```python
from build123d import *

# Parameters (mm, degrees)
BOSS_EXTRUDE1_DEPTH = 40
SKETCH3_R           = 2.5
CUT_EXTRUDE1_DEPTH  = 10
FILLET3_R           = 20


with BuildPart() as part:
    # Sketch1 → Boss-Extrude1 (new body)
    with BuildSketch(Plane.XY):
        Polygon((125.008360384, 233.626853351), (-36.649714989, -46.373146649), (413.350285011, -46.373146649), (413.350285011, 233.626853351), align=None)
        Polygon((393.350285011, 193.626853351), (393.350285011, -16.373146649), (3.764803854, -16.373146649), (125.008360384, 193.626853351), align=None, mode=Mode.SUBTRACT)
    extrude(amount=BOSS_EXTRUDE1_DEPTH)

    # Sketch3 → Cut-Extrude1 (cut)
    with BuildSketch(Plane(origin=(0, 0, 0), x_dir=(-1, 0, 0), z_dir=(0, 0, -1))):
        with Locations((-180.923528507, 226.126853351)):
            Circle(SKETCH3_R)
        with Locations((-200.923528507, 211.126853351)):
            Circle(SKETCH3_R)
        with Locations((-220.923528507, 226.126853351)):
            Circle(SKETCH3_R)
    cut_extrude1 = extrude(amount=-CUT_EXTRUDE1_DEPTH, mode=Mode.SUBTRACT)

    # Mirror1: Cut-Extrude1 across plane
    add(cut_extrude1.mirror(Plane(origin=(264.955285011, 0, 0), x_dir=(0, 0, 1), z_dir=(1, 0, 0))), mode=Mode.SUBTRACT)

    # Fillet3
    fillet3_edges = [part.edges().sort_by_distance(p)[0] for p in [
        (393.350285011, 193.626853351, 20),
        (125.008360384, 193.626853351, 20),
        (3.764803854, -16.373146649, 20),
        (393.350285011, -16.373146649, 20),
        (-36.649714989, -46.373146649, 20),
        (125.008360384, 233.626853351, 20),
        (413.350285011, 233.626853351, 20),
        (413.350285011, -46.373146649, 20),
    ]]
    fillet(fillet3_edges, radius=FILLET3_R)


solid = part.part
```
Check sheet for the modelled part. Datum: model origin and axes. Units: mm. A direction names the side the tool comes from. Round coordinates to 2 decimals unless told otherwise and drop trailing zeros. Loops run counter-clockwise (first coordinate to the right, second up) from the corner with the lowest first, then second, coordinate; pieces in that order, holes last. Notation, with made-up numbers: (-30, 24.5) - (-11, 24.5) arc R28 ccw to (-11, 51.5) - close; hole circle Ø11 at (0.25, 79.25). An arc over 180 degrees is marked (long way). Answer as a JSON object with one key per item and string values. Group by question number.
Q1. Scan lines: line 1 along Y through (x, z) = (335, 27.5); line 2 along X through (y, z) = (53, 8.5); line 3 along X through (y, z) = (181.5, 34.5). Record each from-to range of solid material in increasing order. Write a range as [from, to].
Q2. Sectioned sample at A-A, the plane x = 249.5. Enter the section's corners in (y, z).
Q3. Sectioned sample at B-B, the plane z = 20. Enter the section's corners in (x, y).
Q4. Mould release check, pull along X, two halves, no side actions. Record for faces 3 (the face through (387.647, -10.359, 20.28)), 4 (the face through (193, -46.373, 20)), 5 (the face through (407.34, 227.92, 20.28)): released by +X, released by -X, zero draft, split by the parting line, or undercut.
Q5. Gauge pin test, flat ends, axial feed: P1, Ø4.5, axis at x = 200.92, y = 211.13, coming from the -Z side; P2, Ø1, axis at y = 149, z = 14.5, coming from the -X side; P3, Ø12, axis at y = 58.5, z = 26, coming from the -X side. Record the tip position at first contact, or that the pin passes through.
Q6. Set-up check for faces 1 (the face through (211, -20, 40)), 2 (the face through (387.34, 187.92, 20.28)): record each of +Z, -Z, +X, -X, +Y, -Y from which the full face is reachable in a straight line by a thin tool's end or side.
Q7. Sectioned sample at C-C, the plane y = 8. Enter the section's corners in (x, z).
Solution:
{
 "1": {"line 1": "y = [-46.37, -16.37], [193.63, 233.63]", "line 2": "x = [20.72, 43.82], [393.35, 413.35]", "line 3": "x = [94.91, 118.01], [391.74, 413.35]"},
 "2": {"outline": "(-46.37, 0) - (-16.37, 0) - (-16.37, 40) - (-46.37, 40) - close; (193.63, 0) - (233.63, 0) - (233.63, 40) - (193.63, 40) - close"},
 "3": {"outline": "(-19.33, -16.37) arc R20 ccw to (-2.01, -46.37) - (393.35, -46.37) arc R20 ccw to (413.35, -26.37) - (413.35, 213.63) arc R20 ccw to (393.35, 233.63) - (136.56, 233.63) arc R20 ccw to (119.23, 223.63) - close; hole (21.09, 13.63) arc R20 ccw to (38.41, -16.37) - (373.35, -16.37) arc R20 ccw to (393.35, 3.63) - (393.35, 173.63) arc R20 ccw to (373.35, 193.63) - (136.56, 193.63) arc R20 ccw to (119.23, 183.63) - close"},
 "4": {"face 3": "undercut", "face 4": "zero draft", "face 5": "released by +X"},
 "5": {"P1": "stops at z = 10", "P2": "stops at x = 75.86", "P3": "stops at x = 20.43"},
 "6": {"face 1": "+Z, +X, -X, +Y, -Y", "face 2": "+Z, -Z"},
 "7": {"outline": "(-5.26, 0) - (18.89, 0) - (18.89, 40) - (-5.26, 40) - close; (393.35, 0) - (413.35, 0) - (413.35, 40) - (393.35, 40) - close"}
}
